Input: part model. Units: mm. Frame: model coordinates. Face numbers are marked on the shaded views. A direction names the side the tool comes from. Round coordinates to 2 decimals unless told otherwise and drop trailing zeros. Loops run counter-clockwise (first coordinate to the right, second up) from the corner with the lowest first, then second, coordinate; pieces in that order, holes last. Notation, with made-up numbers: (-29.75, 2) - (23.25, 2) arc R30 cw to (23.25, 29) - close; hole circle Ø3 at (-6.5, 1). An arc over 180 degrees is marked (long way). One line per question, with ' | ' between items. Start each with the question number.
Item 1: Material intervals for line 1 along Z through (x, y) = (0, -15); line 2 along Y through (x, z) = (-6, -9); line 3 along Z through (x, y) = (14, 44), sorted ascending.
Item 2: Set-up query: the marked faces 4, 5 and 6. Return all of +Z, -Z, +X, -X, +Y, -Y with unobstructed straight access to the full face (end or side cutting, diameter ignored); none if empty.
Item 3: Draft query along Z for the marked faces 1, 2 and 3. Return one class per face: pulls with the +Z half, pulls with the -Z half, needs draft (parallel to the pull), parting line crosses it, or undercut.
Item 4: First-contact query: pin 1 (2.5 mm diameter, centred on y = -77.5, z = 0, fed in from -X); pin 2 (9.5 mm diameter, centred on y = -79.5, z = -1, fed in from +X); pin 3 (1.5 mm diameter, centred on x = -2, z = -8, fed in from +Y); pin 4 (10 mm diameter, centred on y = 13, z = 5, fed in from +X). Flat tips, straight axial feed; report the tip coordinate or a pass-through.
Item 5: Section B-B, the plane y = -26. Return loops of the section in (x, z), plus the area to 3 significant figures.
Item 6: Section A-A, the plane y = -68. Return loops of the section in (x, z).
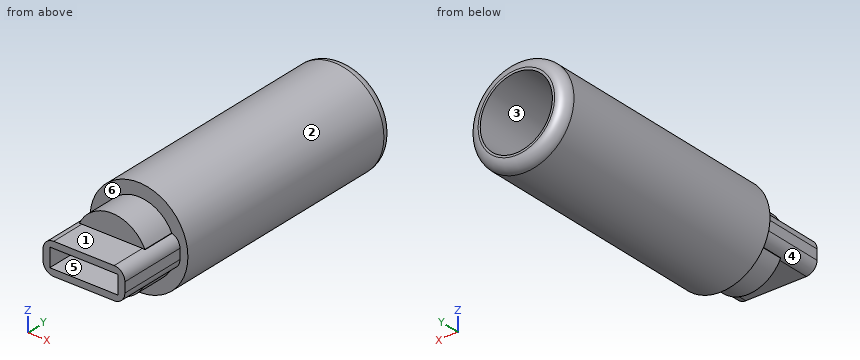
```python
from build123d import *

# Parameters (mm, degrees)
F0_R         = 23.2504682004
F0_R_2       = 17.1266274378
F1_DEPTH     = 59.944
F2_R         = 5.08
F4_W         = 32.4101708829
F4_H         = 8.7824892253
F5_DEPTH     = 32.258
F6_W         = 31.7728198101
F6_H         = 11.3427176839
F6_W_2       = 31.0806287388
F6_H_2       = 14.8886315292
F7_DEPTH     = 16.51
F8_T4_DEPTH  = 57.658
F8_T9_DEPTH  = 44.958
F8_S10_R     = 17.2448690912
F8_T11_DEPTH = 24
F8_T15_DEPTH = 44.958
F8_S16_R     = 17.2448690912
F8_T17_DEPTH = 24
F8_T21_DEPTH = 57.658
F8_T26_DEPTH = 44.958
F8_S27_R     = 17.2448690912
F8_T28_DEPTH = 24
F8_T32_DEPTH = 57.658
F8_T37_DEPTH = 44.958
F8_S38_R     = 17.2448690912
F8_T39_DEPTH = 24
F8_T43_DEPTH = 57.658


# Not quite as in the source:
# - a fillet or chamfer that OpenCascade refuses, or shapes differently, is made with other operations: its cross-section is extruded or revolved along the edge and cut away or added


with BuildPart() as f1:
    # F0 (on Front) → F1 (new body, symmetric)
    with BuildSketch(Plane.XZ):
        with Locations((-0.0308285998, 0.0824332965)):
            Circle(F0_R)
        Circle(F0_R_2, mode=Mode.SUBTRACT)
    extrude(amount=F1_DEPTH, both=True)

    # F2
    f2_edges = [f1.edges().sort_by_distance(p)[0] for p in [
        (-23.281297, 59.944, 0.082433),
    ]]
    fillet(f2_edges, radius=F2_R)

    # F4 (on face) → F5 (join)
    with BuildSketch(Plane.XZ.offset(59.944)):
        Polygon((-15.5403143694, 7.475569495), (-19.4364797935, 7.475569495), (-19.4364797935, -7.475569495), (-15.5403143694, -7.475569495), (15.5403143694, -7.475569495), (19.4364797935, -7.475569495), (19.4364797935, 7.475569495), (15.5403143694, 7.475569495), align=None)
        Rectangle(F4_W, F4_H, mode=Mode.SUBTRACT)
        with BuildLine():
            ThreePointArc((15.5403143694, 7.475569495), (0, 17.2448690912), (-15.5403143694, 7.475569495))
            Line((-15.5403143694, 7.475569495), (15.5403143694, 7.475569495))
        make_face()
        with BuildLine():
            Line((15.5403143694, -7.475569495), (-15.5403143694, -7.475569495))
            ThreePointArc((-15.5403143694, -7.475569495), (0, -17.2448690912), (15.5403143694, -7.475569495))
        make_face()
    extrude(amount=F5_DEPTH)

    # F6 (on face) → F7 (cut)
    with BuildSketch(Plane.XZ.offset(92.202)):
        with Locations((0.3460955357, 13.1469283369)):
            Rectangle(F6_W, F6_H)
        with Locations((0, -14.9198852596)):
            Rectangle(F6_W_2, F6_H_2)
    extrude(amount=-F7_DEPTH, mode=Mode.SUBTRACT)

    # F8: fillet of radius 5.08 on 4 edges, made by hand


with BuildPart() as f8_tool2:
    # F8_s3 → F8_t4 (new body)
    with BuildSketch(Plane.XZ.offset(47.244)):
        with BuildLine():
            ThreePointArc((-14.3564797935, -7.475569495), (-17.9485822419, -5.9876719434), (-19.4364797935, -2.395569495))
            Line((-19.4364797935, -2.395569495), (-19.4364797935, -7.475569495))
            Line((-19.4364797935, -7.475569495), (-14.3564797935, -7.475569495))
        make_face()
    extrude(amount=F8_T4_DEPTH)

    split(bisect_by=Plane.XZ.offset(75.692), keep=Keep.TOP)


with BuildPart() as f1_1:
    add(f1.part)

    # F8_t1: cut F8_tool2
    add(f8_tool2.part, mode=Mode.SUBTRACT)


with BuildPart() as f8_tool7:
    # F8_s8 → F8_t9 (new body)
    with BuildSketch(Plane.XZ.offset(59.944)):
        with BuildLine():
            ThreePointArc((-14.3564797935, -7.475569495), (-17.9485822419, -5.9876719434), (-19.4364797935, -2.395569495))
            Line((-19.4364797935, -2.395569495), (-19.4364797935, -7.475569495))
            Line((-19.4364797935, -7.475569495), (-14.3564797935, -7.475569495))
        make_face()
    extrude(amount=F8_T9_DEPTH)

    # F8_s10 → F8_t11 (cut, symmetric)
    with BuildSketch(Plane.XZ.offset(82.4)):
        Circle(F8_S10_R)
    extrude(amount=F8_T11_DEPTH, both=True, mode=Mode.SUBTRACT)


with BuildPart() as f1_2:
    add(f1_1.part)

    # F8_t6: cut F8_tool7
    add(f8_tool7.part, mode=Mode.SUBTRACT)


with BuildPart() as f8_tool13:
    # F8_s14 → F8_t15 (new body)
    with BuildSketch(Plane.XZ.offset(59.944)):
        with BuildLine():
            ThreePointArc((19.4364797935, -2.395569495), (17.9485822419, -5.9876719434), (14.3564797935, -7.475569495))
            Line((14.3564797935, -7.475569495), (19.4364797935, -7.475569495))
            Line((19.4364797935, -7.475569495), (19.4364797935, -2.395569495))
        make_face()
    extrude(amount=F8_T15_DEPTH)

    # F8_s16 → F8_t17 (cut, symmetric)
    with BuildSketch(Plane.XZ.offset(82.4)):
        Circle(F8_S16_R)
    extrude(amount=F8_T17_DEPTH, both=True, mode=Mode.SUBTRACT)


with BuildPart() as f1_3:
    add(f1_2.part)

    # F8_t12: cut F8_tool13
    add(f8_tool13.part, mode=Mode.SUBTRACT)


with BuildPart() as f8_tool19:
    # F8_s20 → F8_t21 (new body)
    with BuildSketch(Plane.XZ.offset(47.244)):
        with BuildLine():
            ThreePointArc((19.4364797935, -2.395569495), (17.9485822419, -5.9876719434), (14.3564797935, -7.475569495))
            Line((14.3564797935, -7.475569495), (19.4364797935, -7.475569495))
            Line((19.4364797935, -7.475569495), (19.4364797935, -2.395569495))
        make_face()
    extrude(amount=F8_T21_DEPTH)

    split(bisect_by=Plane.XZ.offset(75.692), keep=Keep.TOP)


with BuildPart() as f1_4:
    add(f1_3.part)

    # F8_t18: cut F8_tool19
    add(f8_tool19.part, mode=Mode.SUBTRACT)


with BuildPart() as f8_tool24:
    # F8_s25 → F8_t26 (new body)
    with BuildSketch(Plane.XZ.offset(59.944)):
        with BuildLine():
            ThreePointArc((19.4364797935, 2.395569495), (17.9485822419, 5.9876719434), (14.3564797935, 7.475569495))
            Line((14.3564797935, 7.475569495), (19.4364797935, 7.475569495))
            Line((19.4364797935, 7.475569495), (19.4364797935, 2.395569495))
        make_face()
    extrude(amount=F8_T26_DEPTH)

    # F8_s27 → F8_t28 (cut, symmetric)
    with BuildSketch(Plane.XZ.offset(82.4)):
        Circle(F8_S27_R)
    extrude(amount=F8_T28_DEPTH, both=True, mode=Mode.SUBTRACT)


with BuildPart() as f1_5:
    add(f1_4.part)

    # F8_t23: cut F8_tool24
    add(f8_tool24.part, mode=Mode.SUBTRACT)


with BuildPart() as f8_tool30:
    # F8_s31 → F8_t32 (new body)
    with BuildSketch(Plane.XZ.offset(47.244)):
        with BuildLine():
            ThreePointArc((19.4364797935, 2.395569495), (17.9485822419, 5.9876719434), (14.3564797935, 7.475569495))
            Line((14.3564797935, 7.475569495), (19.4364797935, 7.475569495))
            Line((19.4364797935, 7.475569495), (19.4364797935, 2.395569495))
        make_face()
    extrude(amount=F8_T32_DEPTH)

    split(bisect_by=Plane.XZ.offset(75.692), keep=Keep.TOP)


with BuildPart() as f1_6:
    add(f1_5.part)

    # F8_t29: cut F8_tool30
    add(f8_tool30.part, mode=Mode.SUBTRACT)


with BuildPart() as f8_tool35:
    # F8_s36 → F8_t37 (new body)
    with BuildSketch(Plane.XZ.offset(59.944)):
        with BuildLine():
            ThreePointArc((-19.4364797935, 2.395569495), (-17.9485822419, 5.9876719434), (-14.3564797935, 7.475569495))
            Line((-14.3564797935, 7.475569495), (-19.4364797935, 7.475569495))
            Line((-19.4364797935, 7.475569495), (-19.4364797935, 2.395569495))
        make_face()
    extrude(amount=F8_T37_DEPTH)

    # F8_s38 → F8_t39 (cut, symmetric)
    with BuildSketch(Plane.XZ.offset(82.4)):
        Circle(F8_S38_R)
    extrude(amount=F8_T39_DEPTH, both=True, mode=Mode.SUBTRACT)


with BuildPart() as f1_7:
    add(f1_6.part)

    # F8_t34: cut F8_tool35
    add(f8_tool35.part, mode=Mode.SUBTRACT)


with BuildPart() as f8_tool41:
    # F8_s42 → F8_t43 (new body)
    with BuildSketch(Plane.XZ.offset(47.244)):
        with BuildLine():
            ThreePointArc((-19.4364797935, 2.395569495), (-17.9485822419, 5.9876719434), (-14.3564797935, 7.475569495))
            Line((-14.3564797935, 7.475569495), (-19.4364797935, 7.475569495))
            Line((-19.4364797935, 7.475569495), (-19.4364797935, 2.395569495))
        make_face()
    extrude(amount=F8_T43_DEPTH)

    split(bisect_by=Plane.XZ.offset(75.692), keep=Keep.TOP)


with BuildPart() as f1_8:
    add(f1_7.part)

    # F8_t40: cut F8_tool41
    add(f8_tool41.part, mode=Mode.SUBTRACT)


solid = f1_8.part
```
Return value:
1) line 1: -23.17 to -17.13, 17.13 to 23.33 | line 2: -75.69 to -59.94 | line 3: -18.46 to -9.87, 9.87 to 18.62
2) face 4: -Z, -X, -Y | face 5: +Y, -Y | face 6: -Y
3) face 1: pulls with the +Z half | face 2: parting line crosses it | face 3: undercut
4) pin 1: x = -19.44 | pin 2: x = 19.44 | pin 3: y = -59.94 | pin 4: x = 23.22
5) outline: circle Ø46.5 at (-0.03, 0.08); hole circle Ø34.25 at (0, 0) | area: 777 mm2
6) outline: (-19.44, -2.4) arc R5.08 ccw to (-15.62, -7.32) arc R17.24 ccw to (15.62, -7.32) arc R5.08 ccw to (19.44, -2.4) - (19.44, 2.4) arc R5.08 ccw to (15.62, 7.32) arc R17.24 ccw to (-15.62, 7.32) arc R5.08 ccw to (-19.44, 2.4) - close; hole (-16.21, -4.39) - (16.21, -4.39) - (16.21, 4.39) - (-16.21, 4.39) - close
